```python
from build123d import *

# Parameters (mm, degrees)
SKETCH4_R           = 17.36725
BOSS_EXTRUDE1_DEPTH = 85.725


with BuildPart() as part:
    # Sketch1 → Revolve1 (revolve)
    with BuildSketch(Plane(origin=(0, 0, 0), x_dir=(0, 0, -1), z_dir=(1, 0, 0))):
        Polygon((-57.15, 76.2), (-57.15, 133.35), (57.15, 133.35), (57.15, 76.2), (19.05, 76.2), (19.05, 0), (-19.05, 0), (-19.05, 76.2), align=None)
    revolve(axis=Axis((0, 0, 19.05), (0, 0, -1)))

    # Sketch4 → Boss-Extrude1 (add, symmetric)
    with BuildSketch(Plane(origin=(0, 0, 0), x_dir=(-1, 0, 0), z_dir=(0, 0, -1))):
        Circle(SKETCH4_R)
    extrude(amount=BOSS_EXTRUDE1_DEPTH, both=True)


solid = part.part
```
Part model, mm, in its own coordinate system. A direction names the side the tool comes from. Round coordinates to 2 decimals unless told otherwise and drop trailing zeros. Loops run counter-clockwise (first coordinate to the right, second up) from the corner with the lowest first, then second, coordinate; pieces in that order, holes last. Notation, with made-up numbers: (-9.75, -4.75) -> (5.25, -4.75) arc R14 cw to (5.25, 11.25) -> close; hole circle Ø1 at (-6.5, -7.75). An arc over 180 degrees is marked (long way). Use one line per item in the form item = value. Start each with the question number.
Item 1: Band-saw the part on D-D (z = -70.5). List the corners of the cut face in (x, y).
Item 2: Drop flat-ended pins along their axis: pin 1 Ø3 at (x, y) = (-18, 20) entering from -Z; pin 2 Ø8 at (x, y) = (69.5, 8) entering from +Z; pin 3 Ø8 at (y, z) = (-62, -53) entering from -X. Give the stop position or say it passes through.
Item 3: Two-plate mould, pull along Y, no slides. Class faces 4 (the cylindrical face through (-16.565, 5.217, -52.854)), 5 (the flat face through (0, 0, 85.725)), 6 (the cylindrical face through (40.055, 127.192, -0.8)): released by +Y, released by -Y, zero draft, split by the parting line, or undercut.
Item 4: Tool access for faces 1 (the cylindrical face through (-46.367, -60.47, -37.833)), 2 (the flat face through (0, 0, -85.725)), 3 (the flat face through (18, 1, 19.05)): list every direction of +Z, -Z, +X, -X, +Y, -Y with a clear straight run to the whole face (end or side of a thin tool).
Item 5: Band-saw the part on A-A (x = 0). List the corners of the cut face in (y, z) (3 decimals), plus the area to 3 significant figures.
Item 6: Drill centre lines: line 1 along Y through (x, z) = (70, -44.5); line 2 along Z through (x, y) = (122.5, 32.5); line 3 along Z through (x, y) = (-51, 46.5). Where is each one in solid material? Low to high.
Item 7: Band-saw the part on B-B (z = -26.5). List the corners of the cut face in (x, y), plus the area to 3 significant figures.
Data:
q1.outline = circle Ø34.73 at (0, 0)
q2.pin_1 = -19.05
q2.pin_2 = 19.05
q2.pin_3 = -120.08
q3.face_4 = undercut
q3.face_5 = zero draft
q3.face_6 = split by the parting line
q4.face_1 = -Z
q4.face_2 = -Z, +X, -X, +Y, -Y
q4.face_3 = +Z
q5.outline = (-133.35, -57.15) -> (-76.2, -57.15) -> (-76.2, -19.05) -> (-17.367, -19.05) -> (-17.367, -85.725) -> (17.367, -85.725) -> (17.367, -19.05) -> (76.2, -19.05) -> (76.2, -57.15) -> (133.35, -57.15) -> (133.35, 57.15) -> (76.2, 57.15) -> (76.2, 19.05) -> (17.367, 19.05) -> (17.367, 85.725) -> (-17.367, 85.725) -> (-17.367, 19.05) -> (-76.2, 19.05) -> (-76.2, 57.15) -> (-133.35, 57.15) -> close
q5.area = 23,500 mm^2
q6.line_1 = -113.5 to -30.11, 30.11 to 113.5
q6.line_2 = -57.15 to 57.15
q6.line_3 = -19.05 to 19.05
q7.outline = circle Ø266.7 at (0, 0); circle Ø34.73 at (0, 0); hole circle Ø152.4 at (0, 0)
q7.area = 38,600 mm^2
